The model under review builds one solid part; all positions refer to its coordinate system, in mm. Face numbers are marked on the shaded views. A direction names the side the tool comes from. Round coordinates to 2 decimals unless told otherwise and drop trailing zeros. Order: outer loops, then holes, each group sorted by start corner. A loop starts at its lowest first (then second) coordinate and runs counter-clockwise, first axis right, second up.
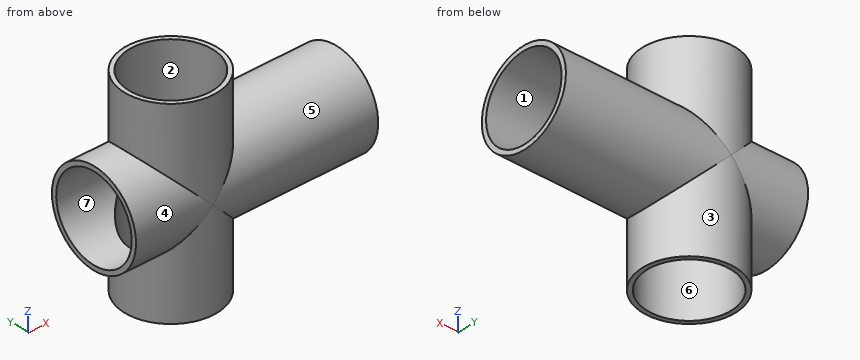
Autodesk Inventor part; units mm, degrees
ref_plane "XZ Plane" through (0, 0, 0) normal (0, 1, 0) x (-1, 0, 0)
ref_plane "XY Plane" through (0, 0, 0) normal (0, 0, 1) x (1, 0, 0)
sketch "Boceto1" plane through (0, 0, 0) normal (0, 0, 1) x (1, 0, 0)
  circle A0 centre (0, 0) radius 95
  dimension "d0" = 190
extrude "Extrusión1" add sketch "Boceto1" along normal blind 400
sketch "Boceto2" plane through (0, 0, 400) normal (0, 0, 1) x (1, 0, 0)
  point P0 (0, 0)
sketch "Boceto3" plane through (0, 0, 400) normal (0, 0, 1) x (1, 0, 0)
  circle A0 centre (0, 0) radius 86.0432
extrude "Extrusión2" cut sketch "Boceto3" against normal blind 400
ref_plane "Plano de trabajo2" through (91.25, 0, 0) normal (1, 0, 0) x (0, 1, 0)
sketch "Boceto4" plane through (91.25, 0, 0) normal (1, 0, 0) x (0, 1, 0)
  line L0 (95, 400) -> (-95, 400) construction
  line L1 (0, 400) -> (0, 0) construction
  line L2 (0, 0) -> (0, 400) construction
  line L3 (0, 400) -> (0, 200) construction
  line L4 (95, 0) -> (95, 400) construction
  line L5 (95, 203.9147) -> (-95, 203.9147) construction
  line L6 (-95, 0) -> (-95, 400) construction
  circle A0 centre (0, 200) radius 95
  dimension "d7" = 190
extrude "Extrusión3" add sketch "Boceto4" along normal mid plane 500
sketch "Boceto5" plane through (0, 0, 400) normal (0, 0, 1) x (1, 0, 0)
  circle A0 centre (0, 0) radius 85.3099
extrude "Extrusión4" cut sketch "Boceto5" against normal blind 500
sketch "Boceto6" plane through (341.25, 0, 200) normal (1, 0, 0) x (0, 0, -1)
  circle A0 centre (0, 0) radius 85.3099
  line L0 (-41.7999, 85.3099) -> (41.7999, 85.3099)
  point P0 (200, 0)
extrude "Extrusión5" cut sketch "Boceto6" against normal blind 500
(1) Consider section B-B (y = 0). State how many separate pieces and enclosed holes the cut face has, and give its area (3 significant figures).
Data:
separate pieces: 4
enclosed holes: 0
area: 10,100 mm2
(2) Insertion check: pin 1 (8 mm diameter, centred on x = 40, z = 258.5, fed in from -Y); pin 2 (6 mm diameter, centred on x = 123.5, y = 67, fed in from +Z); pin 3 (1 mm diameter, centred on x = 257.5, z = 184.5, fed in from +Y). Each pin has a flat end and moves straight along its axis. Give the tip position at first contact, or say it passes through.
Data:
pin 1: stops at y = -87.91
pin 2: stops at z = 270.21
pin 3: stops at y = 93.81
(3) For the marked faces 1, 2, 3 and 4, list the 3-axis set-ups (+Z, -Z, +X, -X, +Y, -Y) from which the entire face can be reached by the end or side of a thin tool; tool diameter is ignored.
Data:
face 1: +X, -X
face 2: +Z
face 3: -Z
face 4: -X
(4) Consider section A-A (z = 230). Write out the cut boundary in (x, y), and give its area (3 significant figures).
Data:
outline: (-158.75, -90.14) - (-30, -90.14) arc R95 ccw to (30, -90.14) - (341.25, -90.14) - (341.25, -79.86) - (30, -79.86) arc R85.31 cw to (-30, -79.86) - (-158.75, -79.86) - close; (-158.75, 79.86) - (-30, 79.86) arc R85.31 cw to (30, 79.86) - (341.25, 79.86) - (341.25, 90.14) - (30, 90.14) arc R95 ccw to (-30, 90.14) - (-158.75, 90.14) - close
area: 10,200 mm2
(5) Consider section C-C (x = 70.5). Write out the cut boundary in (y, z), and give its area (3 significant figures).
Data:
outline: (-63.68, 0) - (-49.33, 0) - (-49.33, 118.81) arc R95 ccw to (-48.04, 118.04) - (-48.04, 129.5) arc R85.31 cw to (-48.04, 270.5) - (-48.04, 281.96) arc R95 ccw to (-49.33, 281.19) - (-49.33, 400) - (-63.68, 400) - (-63.68, 270.5) arc R95 ccw to (-63.68, 129.5) - close; (48.04, 118.04) arc R95 ccw to (49.33, 118.81) - (49.33, 0) - (63.68, 0) - (63.68, 129.5) arc R95 ccw to (63.68, 270.5) - (63.68, 400) - (49.33, 400) - (49.33, 281.19) arc R95 ccw to (48.04, 281.96) - (48.04, 270.5) arc R85.31 cw to (48.04, 129.5) - close
area: 10,600 mm2
(6) Consider section D-D (z = 138.5). Write out the cut boundary in (x, y).
Data:
outline: (-158.75, -72.41) - (-61.5, -72.41) arc R95 ccw to (61.5, -72.41) - (341.25, -72.41) - (341.25, -59.12) - (61.5, -59.12) arc R85.31 cw to (45.11, -72.41) - (46.48, -72.41) arc R86.04 cw to (-46.48, -72.41) - (-45.11, -72.41) arc R85.31 cw to (-61.5, -59.12) - (-158.75, -59.12) - close; (-158.75, 59.12) - (-61.5, 59.12) arc R85.31 cw to (-45.11, 72.41) - (-46.48, 72.41) arc R86.04 cw to (46.48, 72.41) - (45.11, 72.41) arc R85.31 cw to (61.5, 59.12) - (341.25, 59.12) - (341.25, 72.41) - (61.5, 72.41) arc R95 ccw to (-61.5, 72.41) - (-158.75, 72.41) - close
(7) Draft analysis for pull direction Z (two halves, no side actions). For the marked faces 5, 6 and 7, state which applies: pulls with the +Z half, pulls with the -Z half, needs draft (parallel to the pull), parting line crosses it, or undercut.
Data:
face 5: parting line crosses it
face 6: needs draft
face 7: undercut
(8) To check wall thickness, follow probe 1 along Y at (x, z) = (0, 244.5); probe 2 along Y at (x, z) = (125.5, 200). State the ranges of each line that lie inside material, in increasing order.
Data:
probe 1: y = -95 to -86.04, 86.04 to 95
probe 2: y = -95 to -85.31, 85.31 to 95
